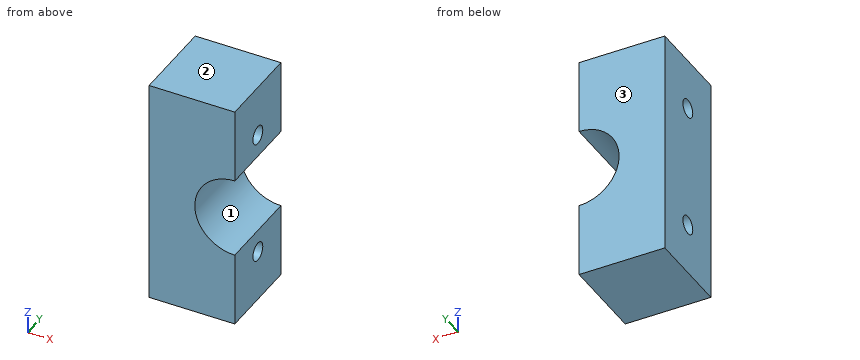
from build123d import *

# Parameters (mm, degrees)
BOSS_EXTRUDE1_DEPTH = 15
CUT_EXTRUDE2_REACH  = 17
SKETCH4_R           = 1.6


with BuildPart() as part:
    # Sketch1 → Boss-Extrude1 (new body)
    with BuildSketch(Plane(origin=(0, 0, 0), x_dir=(1, 0, 0), z_dir=(0, 1, 0))):
        with BuildLine():
            Line((7.5, 20), (7.5, 7))
            ThreePointArc((7.5, 7), (0.5, 0), (7.5, -7))
            Line((7.5, -7), (7.5, -20))
            Line((7.5, -20), (-7.5, -20))
            Line((-7.5, -20), (-7.5, 20))
            Line((-7.5, 20), (7.5, 20))
        make_face()
    extrude(amount=BOSS_EXTRUDE1_DEPTH)

    # Sketch4 → Cut-Extrude2 (cut, up to next)
    with BuildSketch(Plane(origin=(7.5, 0, 0), x_dir=(0, 0, -1), z_dir=(1, 0, 0)), mode=Mode.PRIVATE) as cut_extrude2_sk1:
        with Locations((11, 7.5)):
            Circle(SKETCH4_R)
    cut_extrude2_tool1 = extrude(cut_extrude2_sk1.sketch, amount=-CUT_EXTRUDE2_REACH, mode=Mode.PRIVATE) & part.part
    add(cut_extrude2_tool1.solids().sort_by_distance((7.5, 7.5, -11))[0], mode=Mode.SUBTRACT)
    # Sketch4 → Cut-Extrude2 (cut, up to next)
    with BuildSketch(Plane(origin=(7.5, 0, 0), x_dir=(0, 0, -1), z_dir=(1, 0, 0)), mode=Mode.PRIVATE) as cut_extrude2_sk2:
        with Locations((-11, 7.5)):
            Circle(SKETCH4_R)
    cut_extrude2_tool2 = extrude(cut_extrude2_sk2.sketch, amount=-CUT_EXTRUDE2_REACH, mode=Mode.PRIVATE) & part.part
    add(cut_extrude2_tool2.solids().sort_by_distance((7.5, 7.5, 11))[0], mode=Mode.SUBTRACT)


solid = part.part
Read the model definition and answer for the solid it produces. Units are mm, in the model's axes. Face numbers are marked on the shaded views. Round coordinates to 2 decimals unless told otherwise and drop trailing zeros. Write each loop counter-clockwise with the first axis right and the second up, starting at its lowest first coordinate (ties: lowest second). Pieces come first, ordered by that corner, then holes. Notation, with made-up numbers: (-32, 7) - (-28, 7) arc R10 cw to (-28, 18) - close; hole circle Ø1 at (18, 33). An arc over 180 degrees is marked (long way). One line per question, with ' | ' between items. Start each with the question number.
1. For a pull along Z with two mould halves and no side action, classify the marked faces 1, 2 and 3 as +Z half, -Z half, draft (parallel to the pull), parting line (faces both ways), or undercut.
2. Find the intervals of material crossed by probe 1 along Y at (x, z) = (-3, -11); probe 2 along Z at (x, y) = (-3.5, 7.25); probe 3 along X at (y, z) = (12.75, 0), in increasing order. Write a range as [from, to].
3. Section C-C (y = 7.5) is taken. Determine the outline of the cut face in (x, z).
4. Section D-D (x = -1.25) is taken. Determine the outline of the cut face in (y, z).
5. Section B-B (x = 5.5) is taken. Determine the outline of the cut face in (y, z), and give its area (3 significant figures).
6. Each of these flat-tipped pins is pushed along its axis until it touches: pin 1 (6 mm diameter, centred on x = 5.5, z = -0.5, fed in from +Y); pin 2 (4 mm diameter, centred on y = 7.5, z = -11, fed in from +X); pin 3 (1.5 mm diameter, centred on y = 12, z = 1, fed in from +X). Where does it stop, or does it pass through?
7. Section A-A (z = 11) is taken. Determine the outline of the cut face in (x, y), and give its area (3 significant figures).
Filled in:
1) face 1: undercut | face 2: +Z half | face 3: draft
2) probe 1: [0, 5.9], [9.1, 15] | probe 2: [-20, -12.58], [-9.42, 9.42], [12.58, 20] | probe 3: [-7.5, 0.5]
3) outline: (-7.5, -20) - (7.5, -20) - (7.5, -12.6) - (-7.5, -12.6) - close; (-7.5, -9.4) - (7.5, -9.4) - (7.5, -7) arc R7 cw to (7.5, 7) - (7.5, 9.4) - (-7.5, 9.4) - close; (-7.5, 12.6) - (7.5, 12.6) - (7.5, 20) - (-7.5, 20) - close
4) outline: (0, -20) - (15, -20) - (15, 20) - (0, 20) - close; hole circle Ø3.2 at (7.5, -11); hole circle Ø3.2 at (7.5, 11)
5) outline: (0, -20) - (15, -20) - (15, -6.71) - (0, -6.71) - close; (0, 6.71) - (15, 6.71) - (15, 20) - (0, 20) - close; hole circle Ø3.2 at (7.5, -11); hole circle Ø3.2 at (7.5, 11) | area: 383 mm²
6) pin 1: through | pin 2: x = 7.5 | pin 3: x = 0.72
7) outline: (-7.5, 0) - (7.5, 0) - (7.5, 5.9) - (-7.5, 5.9) - close; (-7.5, 9.1) - (7.5, 9.1) - (7.5, 15) - (-7.5, 15) - close | area: 177 mm²
